Part model, mm, in its own coordinate system. A direction names the side the tool comes from. Give positions to 0.01 mm unless a question says otherwise; leave off trailing zeros. Write each loop counter-clockwise with the first axis right and the second up, starting at its lowest first coordinate (ties: lowest second). Pieces come first, ordered by that corner, then holes. Notation, with made-up numbers: (85, -6.75) - (119, -6.75) arc R8 ccw to (119, 7.25) - close; hole circle Ø2 at (-24.5, -12). An arc over 180 degrees is marked (long way). Answer as a JSON object with one key per item and string values. Group by question number.
```python
from build123d import *

# Parameters (mm, degrees)
BOSS_EXTRUDE1_DEPTH = 50
CUT_EXTRUDE1_REACH  = 199.772
SKETCH2_R           = 10


with BuildPart() as part:
    # Sketch1 → Boss-Extrude1 (new, symmetric)
    with BuildSketch(Plane.XY):
        with BuildLine():
            Line((-65.812232905, -73), (-112.886751346, -73))
            Line((-112.886751346, -73), (-112.886751346, -90))
            Line((-112.886751346, -90), (-2.886751346, -90))
            Line((-2.886751346, -90), (-41.13620668, -23.75))
            ThreePointArc((-41.13620668, -23.75), (12.293904642, 45.881476749), (23.75, -41.13620668))
            Line((23.75, -41.13620668), (51.961524227, -90))
            Line((51.961524227, -90), (112.113248654, -90))
            Line((112.113248654, -90), (112.113248654, -73))
            Line((112.113248654, -73), (68.704682034, -73))
            ThreePointArc((68.704682034, -73), (62.704682034, -71.392304845), (58.312377188, -67))
            Line((58.312377188, -67), (45.832116851, -45.383555005))
            ThreePointArc((45.832116851, -45.383555005), (3.304284934, 64.415306419), (-50.235373046, -40.455621302))
            ThreePointArc((-50.235373046, -40.455621302), (-47.772172291, -61.634593969), (-65.812232905, -73))
        make_face()
    extrude(amount=BOSS_EXTRUDE1_DEPTH, both=True)

    # Sketch2 → Cut-Extrude1 (cut, up to next)
    with BuildSketch(Plane.XZ.offset(90), mode=Mode.PRIVATE) as cut_extrude1_sk1:
        with Locations(Location((90, 0, 0), (0, 0, 270))):
            Circle(SKETCH2_R)
    cut_extrude1_tool1 = extrude(cut_extrude1_sk1.sketch, amount=-CUT_EXTRUDE1_REACH, mode=Mode.PRIVATE) & part.part
    # Sketch2 → Cut-Extrude1 (cut, up to next)
    with BuildSketch(Plane.XZ.offset(90), mode=Mode.PRIVATE) as cut_extrude1_sk2:
        with Locations(Location((-90, 0, 0), (0, 0, 270))):
            Circle(SKETCH2_R)
    cut_extrude1_tool2 = extrude(cut_extrude1_sk2.sketch, amount=-CUT_EXTRUDE1_REACH, mode=Mode.PRIVATE) & part.part
    add(cut_extrude1_tool1.solids().sort_by_distance((90, -90, 0))[0], mode=Mode.SUBTRACT)
    add(cut_extrude1_tool2.solids().sort_by_distance((-90, -90, 0))[0], mode=Mode.SUBTRACT)


solid = part.part
```
1) Which spindle directions (+Z, -Z, +X, -X, +Y, -Y) get a long thin tool onto all of the face, cutting with end or side? Do faces 5 (the flat face through (-59, -90, 1)), 6 (the flat face through (100.4, -73, 0.7)), 7 (the flat face through (-79, -73, 1)), 8 (the flat face through (52.16, -56.34, 0.7)), 9 (the flat face through (-21.744, -57.339, 0.7)). Say none if no direction does.
2) Band-saw the part on C-C (z = -20). List the corners of the cut face in (x, y).
3) Probe line 1 (X direction, y = -76.75, z = 0); line 2 (X direction, y = 0, z = 27); line 3 (X direction, y = -85, z = 0). List the from-to ranges inside material, lowest first.
4) Band-saw the part on A-A (y = 0). List the corners of the cut face in (x, z), plus the area to 3 significant figures.
5) Band-saw the part on D-D (x = 0). List the corners of the cut face in (y, z), plus the area to 3 significant figures.
6) Drop flat-ended pins along their axis: P1, Ø3, axis at x = 13.5, z = -17.5, coming from the +Y side; P2, Ø1.5, axis at y = -53, z = 28.5, coming from the +X side; P3, Ø1.5, axis at y = -26, z = 9, coming from the +X side. Give the stop position or say it passes through.
7) Band-saw the part on B-B (x = -90). List the corners of the cut face in (y, z), plus the area to 3 significant figures.
8) Mould opens along Z. For faces 1 (the flat face through (-34, -41, -50)), 2 (the cylindrical face through (-80.085, -81.619, 1.302)), 3 (the flat face through (-34, -41, 50)), 4 (the flat face through (37.66, -65.23, 0.7)) say: pulls with the +Z half, pulls with the -Z half, needs draft (parallel to the pull), parting line crosses it, or undercut.
Verdict:
{
 "1": {"face 5": "+Z, -Z, +X, -X, -Y", "face 6": "+Z, -Z, +X, +Y", "face 7": "+Z, -Z, -X, +Y", "face 8": "+Z, -Z, +X", "face 9": "+Z, -Z"},
 "2": {"outline": "(-112.89, -90) - (-2.89, -90) - (-41.14, -23.75) arc R47.5 cw (long way) to (23.75, -41.14) - (51.96, -90) - (112.11, -90) - (112.11, -73) - (68.7, -73) arc R12 cw to (58.31, -67) - (45.83, -45.38) arc R64.5 ccw (long way) to (-50.24, -40.46) arc R20 cw to (-65.81, -73) - (-112.89, -73) - close"},
 "3": {"line 1": "-112.89 to -100, -80 to -10.54, 44.31 to 80, 100 to 112.11", "line 2": "-64.5 to -47.5, 47.5 to 64.5", "line 3": "-112.89 to -100, -80 to -5.77, 49.07 to 80, 100 to 112.11"},
 "4": {"outline": "(-64.5, -50) - (-47.5, -50) - (-47.5, 50) - (-64.5, 50) - close; (47.5, -50) - (64.5, -50) - (64.5, 50) - (47.5, 50) - close", "area": "3,400 mm2"},
 "5": {"outline": "(47.5, -50) - (64.5, -50) - (64.5, 50) - (47.5, 50) - close", "area": "1,700 mm2"},
 "6": {"P1": "y = 63.37", "P2": "x = 50.66", "P3": "x = 59.35"},
 "7": {"outline": "(-90, -50) - (-73, -50) - (-73, -10) - (-90, -10) - close; (-90, 10) - (-73, 10) - (-73, 50) - (-90, 50) - close", "area": "1,360 mm2"},
 "8": {"face 1": "pulls with the -Z half", "face 2": "undercut", "face 3": "pulls with the +Z half", "face 4": "needs draft"}
}
